from build123d import *

# Parameters (mm, degrees)
F1_ANGLE_BACK = 90
F1_ANGLE      = 180
F3_DEPTH      = 119.4722198035
F4_R          = 2


with BuildPart() as f1:
    # F0 (on Front) → F1 (revolve)
    with BuildSketch(Plane.XZ, mode=Mode.PRIVATE) as f1_sk:
        Polygon((-73.7361099018, -26.5), (-69.7183494024, -26.5), (-64.7183494024, 26.5), (-68.7361099018, 26.5), align=None)
    revolve(f1_sk.sketch.rotate(Axis((-59.7361099018, 0, 0), (0, 0, -1)), -F1_ANGLE_BACK), axis=Axis((-59.7361099018, 0, 0), (0, 0, -1)), revolution_arc=F1_ANGLE)


with BuildPart() as f2_1:
    # F2: instance of F1
    add(f1.part.mirror(Plane.YZ))


with BuildPart() as f1_1:
    add(f1.part)

    # F3 (add, through all): faces of the model
    f3_faces = [f1_1.faces().sort_by_distance(p)[0] for p in [
        (-59.7361099018, -9.4911197503, 0),
        (-59.7361099018, 9.4911197503, 0),
    ]]

    add(f2_1.part)  # F3 merges F2_1
    extrude(f3_faces, amount=F3_DEPTH)

    # F4
    f4_edges = [f1_1.edges().sort_by_distance(p)[0] for p in [
        (68.73611, 0, 26.5),
    ]]
    fillet(f4_edges, radius=F4_R)


solid = f1_1.part
For this review, take the finished solid that the model builds, in its own axes (mm). A direction names the side the tool comes from. Round coordinates to 2 decimals unless told otherwise and drop trailing zeros. Loops run counter-clockwise (first coordinate to the right, second up) from the corner with the lowest first, then second, coordinate; pieces in that order, holes last. Notation, with made-up numbers: (9, 44.5) - (16, 44.5) arc R27 cw to (16, 75.5) - close; hole circle Ø1 at (25, 37.5). An arc over 180 degrees is marked (long way). Answer as CSV lines item,"result".
(1) Consider section B-B on y = 0. Give the boundary of the cut face in (x, z).
Checked values:
outline,"(-73.74, -26.5) - (-69.72, -26.5) - (-64.72, 26.5) - (-66.92, 26.5) arc R2 ccw to (-68.91, 24.69) - close; (64.72, 26.5) - (69.72, -26.5) - (73.74, -26.5) - (68.91, 24.69) arc R2 ccw to (66.92, 26.5) - close"
(2) Consider section C-C on z = -14.5. Give the boundary of the cut face in (x, y), then the cut area to 3 significant figures.
Checked values:
outline,"(-59.74, -12.87) - (59.74, -12.87) arc R12.87 ccw to (59.74, 12.87) - (-59.74, 12.87) arc R12.87 ccw to start; hole (-59.74, -8.85) - (59.74, -8.85) arc R8.85 ccw to (59.74, 8.85) - (-59.74, 8.85) arc R8.85 ccw to start"
area,"1,230 mm2"
(3) Consider section D-D on z = -5.5. Give the boundary of the cut face in (x, y).
Checked values:
outline,"(-59.74, -12.02) - (59.74, -12.02) arc R12.02 ccw to (59.74, 12.02) - (-59.74, 12.02) arc R12.02 ccw to start; hole (-59.74, -8) - (59.74, -8) arc R8 ccw to (59.74, 8) - (-59.74, 8) arc R8 ccw to start"
(4) Tool access review of faces 1 (the face through (67.18, -0.16, 0.37)), 2 (the face through (-0.84, 11.55, -0.55)): name each direction out of +Z, -Z, +X, -X, +Y, -Y from which nothing blocks a thin tool from reaching the whole face with its end or side.
Checked values:
face 1,"-Z"
face 2,"+Z, +X, -X, +Y"
(5) Mouldability with a two-part tool opening along Y and no side actions: class faces 3 (the face through (71.353, -0.256, -1.264)), 4 (the face through (-0.3, 10.3, -26.5)), 5 (the face through (-67.18, -0.16, 0.37)) as +Y half, -Y half, draft (parallel to the pull), parting line (faces both ways), or undercut.
Checked values:
face 3,"parting line"
face 4,"draft"
face 5,"undercut"
(6) Wall thickness on line 1 (Y direction, x = 33.5, z = -22.5); line 2 (X direction, y = 6.75, z = 0.5); line 3 (Y direction, x = 63.5, z = -5): over which ranges is each line inside the solid? List them lowest first.
Checked values:
line 1,"y = -13.62 to -9.6, 9.6 to 13.62"
line 2,"x = -68.99 to -62.85, 62.85 to 68.99"
line 3,"y = -11.36 to -7.01, 7.01 to 11.36"
(7) Insertion check: P1, Ø10, axis at x = -44, z = 15, coming from the -Y side; P2, Ø6, axis at x = 23, z = 15.5, coming from the +Y side; P3, Ø2, axis at y = -11, z = -5, coming from the -X side. Each pin has a flat end and moves straight along its axis. Give the tip position at first contact, or say it passes through.
Checked values:
P1,"stops at y = -10.56"
P2,"stops at y = 10.32"
P3,"stops at x = -66.33"
(8) Consider section A-A on x = -11.5. Give the boundary of the cut face in (y, z), then the cut area to 3 significant figures.
Checked values:
outline,"(-14, -26.5) - (-9.98, -26.5) - (-4.98, 26.5) - (-7.18, 26.5) arc R2 ccw to (-9.17, 24.69) - close; (4.98, 26.5) - (9.98, -26.5) - (14, -26.5) - (9.17, 24.69) arc R2 ccw to (7.18, 26.5) - close"
area,"425 mm2"
